Answer from the drawing. Dimensions are ordinates in mm from the lowest x, y and z of the part. Give positions to 0.01 mm unless a question says otherwise; leave off trailing zeros. Order: outer loops, then holes, each group sorted by start corner. A loop starts at its lowest first (then second) coordinate and runs counter-clockwise, first axis right, second up. Notation, with made-up numbers: (27, -8.75) - (46, -8.75) arc R14 ccw to (46, 0.25) - close; hole circle Ø7 at (9, 65.5). An arc over 180 degrees is marked (long way). Answer in a Markdown table with one row per item.
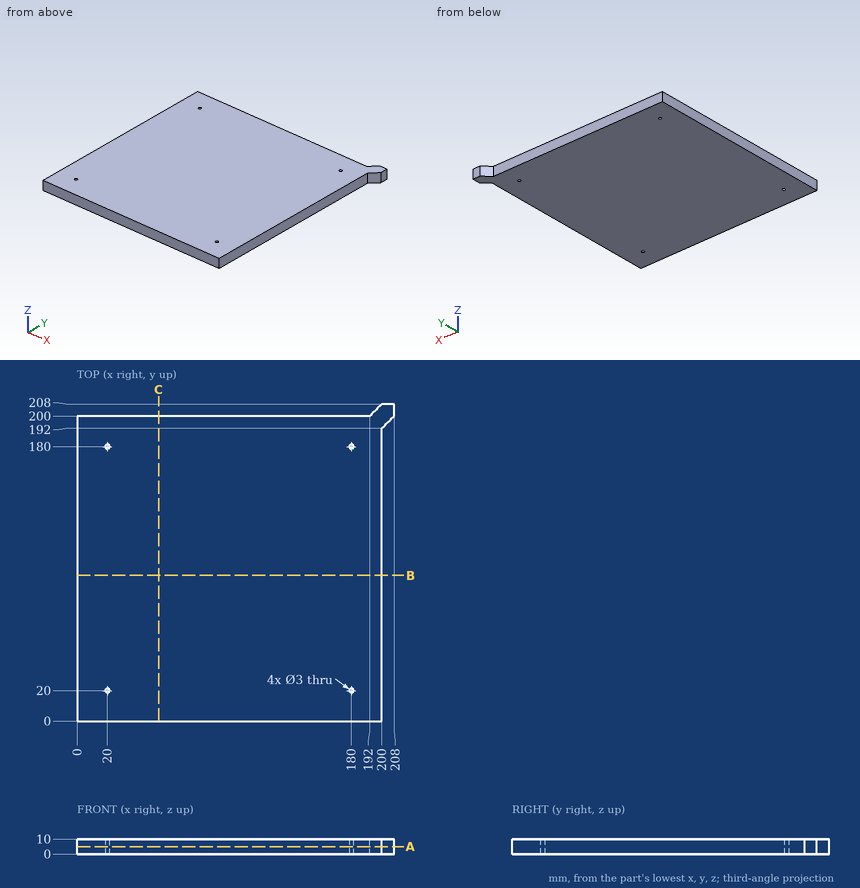
Item 1: Consider line 1 (X direction, y = 180, z = 4); line 2 (X direction, y = 146.5, z = 1.25). Determine where each line is inside the solid, lowest interval first.
Answer block:
| item | result |
|---|---|
| line 1 | 0 to 18.5, 21.5 to 178.5, 181.5 to 200 |
| line 2 | 0 to 200 |
Item 2: Find section B-B on y = 95.5. Write down the section's boundary in (x, z).
Answer block:
| item | result |
|---|---|
| outline | (0, 0) - (200, 0) - (200, 10) - (0, 10) - close |
Item 3: This flat-tipped pin is pushed along its axis until it touches: P1, Ø3, axis at x = 136.5, z = 7.5, coming from the +Y side. Where does it stop, or does it pass through?
Answer block:
| item | result |
|---|---|
| P1 | y = 200 |
Item 4: Find section A-A on z = 5. Write down the section's boundary in (x, y), then the cut area to 3 significant figures.
Answer block:
| item | result |
|---|---|
| outline | (0, 0) - (200, 0) - (200, 192) - (208, 200) - (208, 208) - (200, 208) - (192, 200) - (0, 200) - close; hole circle Ø3 at (20, 20); hole circle Ø3 at (20, 180); hole circle Ø3 at (180, 20); hole circle Ø3 at (180, 180) |
| area | 40,100 mm² |
